Autodesk Inventor part; units mm, degrees
ref_plane "YZ Plane" through (0, 0, 0) normal (1, 0, 0) x (0, 1, 0)
ref_plane "XZ Plane" through (0, 0, 0) normal (0, 1, 0) x (-1, 0, 0)
ref_plane "XY Plane" through (0, 0, 0) normal (0, 0, 1) x (1, 0, 0)
sketch "Sketch1" plane through (0, 0, 0) normal (0, 1, 0) x (-1, 0, 0)
  line L0 (26, 0) -> (-26, 0)
  line L1 (-26, 0) -> (-26, -26)
  line L2 (-26, -26) -> (26, -26)
  line L3 (26, -26) -> (26, 0)
  point P0 (0, 0)
  dimension "d0" = 52
  dimension "d1" = 26
  dimension "d2" = 26
  dimension "d3" = 26
extrude "Extrusion1" add sketch "Sketch1" along normal blind 35
sketch "Sketch3" plane through (-26, 0, 0) normal (0, 0, 1) x (1, 0, 0)
  line L0 (0, 35) -> (52, 35)
  line L1 (38.8, 35) -> (65.2826, 35)
  line L2 (65.2826, 35) -> (65.2826, 0)
  line L3 (26, -13.8937) -> (26, 45.4279)
  line L4 (52, 0) -> (52, 35)
  arc A0 (52, 10.4979) -> (38.8, 35) centre (22.6594, 10.4979) ccw
  line L5 (52, 10.4979) -> (52, 0)
  line L6 (65.2826, 0) -> (52, 0)
  point P0 (26, 0)
  point P1 (52, 10.9288)
  dimension "d7" = 90
  dimension "d33" = 12.8
revolve "Revolution1" cut sketch "Sketch3" angle 360 about axis through (0, 35, 0) along (0, 1, 0)
sketch "Sketch2" plane through (0, 35, 0) normal (0, 1, 0) x (1, 0, 0)
  circle A0 centre (0, 0) radius 12.8
  dimension "d6" = 25.6
extrude "Extrusion2" cut sketch "Sketch2" against normal blind 1
sketch "Sketch4" plane through (0, 34, 0) normal (0, 1, 0) x (1, 0, 0)
  circle A0 centre (0, 0) radius 11.4
  dimension "d11" = 22.8
extrude "Extrusion3" cut sketch "Sketch4" against normal through all
sketch "Sketch5" plane through (0, 0, 0) normal (0, -1, 0) x (1, 0, 0)
  circle A0 centre (0, 0) radius 16.4
  dimension "d16" = 32.8
extrude "Extrusion4" cut sketch "Sketch5" against normal blind 26
sketch "Sketch8" plane through (0, 0, 0) normal (0, -1, 0) x (1, 0, 0)
  circle A0 centre (0, -21) radius 2.7
  point P0 (0, 0)
  dimension "d21" = 5.4
  dimension "d22" = 21
extrude "Extrusion5" add sketch "Sketch8" along normal blind 5
pattern_circular "Circular Pattern1" count 5 over 240 about axis through (0, 35, 0) along (0, 1, 0) of "Extrusion5" both ways yes
mirror "Mirror1" about plane through (-26, 0, 0) normal (0, 0, 1) of "Extrusion4", "Extrusion1", "Revolution1", "Extrusion2", "Extrusion3"
fillet "Fillet2" radius 1 1 edges at (-16.4, 26, 0)
ref_plane "Work Plane1" through (0, 8, 0) normal (0, 1, 0) x (1, 0, 0)
sketch "Sketch10" plane through (0, 8, 0) normal (0, 1, 0) x (1, 0, 0)
  circle A0 centre (0, 0) radius 42.5144
extrude "Extrusion7" cut sketch "Sketch10" along normal blind 40
equation "\"d1\" = 0.5 * d0"
properties part number "_3DPrint"
The listing builds one solid part. Answer for the finished solid, in the listing's coordinates (mm). A direction names the side the tool comes from. Round coordinates to 2 decimals unless told otherwise and drop trailing zeros. Write each loop counter-clockwise with the first axis right and the second up, starting at its lowest first coordinate (ties: lowest second). Pieces come first, ordered by that corner, then holes. Notation, with made-up numbers: M -14,75.25 L 10,75.25 A35 cw 10,108.25 Z; hole C 80.5,-31.75 d7. An arc over 180 degrees is marked long. Write each question's results on one line, items separated by ' | '. Start each with the question number.
Item 1: A cutting plane is placed at A-A on z = 0. Write down the section's boundary in (x, y).
Item 2: Straight lines are drawn through the part: L1, parallel to X at y = 6, z = 0; L2, parallel to Y at x = -15, z = 13.5. For each, find the intervals that lie inside material, in ascending order. Write a range as [from, to].
Item 3: For a pull along Z with two mould halves and no side action, classify faces 1 (the face through (-2.13, 3.94, 16.26)), 2 (the face through (-0.351, -2.465, -23.677)), 3 (the face through (-18, -5, -10)) as pulls with the +Z half, pulls with the -Z half, needs draft (parallel to the pull), parting line crosses it, or undercut.
Item 4: A cutting plane is placed at C-C on y = 2.75. Write down the section's boundary in (x, z).
Item 5: For faces 4 (the face through (-15.61, -2.46, 9.69)), 5 (the face through (18, -5, 10)), determine the directions among +Z, -Z, +X, -X, +Y, -Y from which every point of the face is accessible in a straight line to the end or side of a thin tool.
Item 6: Flat-ended cylindrical pins translate along their axes: pin 1 Ø4 at (y, z) = (3.5, 18) entering from +X; pin 2 Ø3 at (x, y) = (-12.5, -2.5) entering from -Z; pin 3 Ø3 at (y, z) = (2.5, -7) entering from -X; pin 4 Ø2 at (y, z) = (6.5, -20.5) entering from -X. Find the tip coordinate at first contact, or state that the pin passes through.
Item 7: A cutting plane is placed at B-B on x = 0. Write down the section's boundary in (y, z).
Item 8: A cutting plane is placed at D-D on z = -9. Write down the section's boundary in (x, y), and give its area (3 significant figures).
Check sheet entries:
1) outline: M -26,0 L -16.4,0 L -16.4,8 L -26,8 Z; M 16.4,0 L 26,0 L 26,8 L 16.4,8 Z
2) L1: [-26, -16.4], [16.4, 26] | L2: [0, 8]
3) face 1: undercut | face 2: parting line crosses it | face 3: needs draft
4) outline: C 0,0 d52; hole C 0,0 d32.8
5) face 4: -Y | face 5: +Z, -Z, +X, -X, -Y
6) pin 1: x = 20.49 | pin 2: through | pin 3: x = -25.41 | pin 4: x = -17.2
7) outline: M -5,-23.7 L 0,-23.7 L 0,-26 L 8,-26 L 8,-16.4 L 0,-16.4 L 0,-18.3 L -5,-18.3 Z; M 0,16.4 L 8,16.4 L 8,26 L 0,26 Z
8) outline: M -24.39,0 L -20.43,0 L -20.43,-5 L -15.94,-5 L -15.94,0 L -13.71,0 L -13.71,8 L -24.39,8 Z; M 13.71,0 L 15.94,0 L 15.94,-5 L 20.43,-5 L 20.43,0 L 24.39,0 L 24.39,8 L 13.71,8 Z | area: 216 mm²
